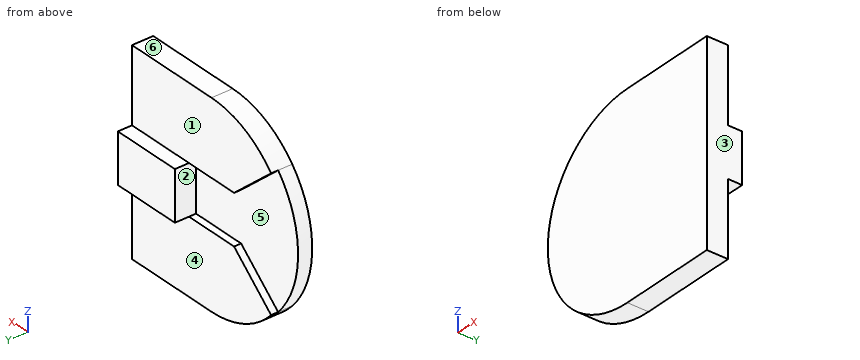
from build123d import *

# Parameters (mm, degrees)
BOSS_EXTRUDE2_DEPTH = 2
BOSS_EXTRUDE3_DEPTH = 3
BOSS_EXTRUDE5_DEPTH = 5


with BuildPart() as part:
    # Sketch1 → Boss-Extrude2 (new body)
    with BuildSketch(Plane(origin=(0, 0, 0), x_dir=(1, 0, 0), z_dir=(0, 1, 0))):
        Polygon((-6.445352893, 3.5), (-10.403887085, 3.5), (-10.403887085, 0), align=None)
        Polygon((-6.445352893, -3.5), (-10.403887085, 0), (-6.445352893, 3.5), (-6.445352893, 0), align=None)
        Polygon((-6.445352893, -3.5), (-10.403887085, 0), (-10.403887085, -3.5), align=None)
        Polygon((-10.403887085, 0), (-10.403887085, 3.5), (-14.362421277, 3.5), align=None)
        with BuildLine():
            Line((-14.362421277, 3.5), (-20.861114748, 9.245921608))
            ThreePointArc((-20.861114748, 9.245921608), (-24.362421277, 0), (-20.861114748, -9.245921608))
            Line((-20.861114748, -9.245921608), (-14.362421277, -3.5))
            Line((-14.362421277, -3.5), (-10.403887085, 0))
            Line((-10.403887085, 0), (-14.362421277, 3.5))
        make_face()
        Polygon((-10.403887085, -3.5), (-10.403887085, 0), (-14.362421277, -3.5), align=None)
    extrude(amount=BOSS_EXTRUDE2_DEPTH)

    # Sketch1_5 → Boss-Extrude3 (add)
    with BuildSketch(Plane(origin=(0, 0, 0), x_dir=(1, 0, 0), z_dir=(0, 1, 0))):
        with BuildLine():
            Line((-10.403887085, 3.5), (-10.403887085, 13.958534192))
            ThreePointArc((-10.403887085, 13.958534192), (-16.138918204, 12.725961451), (-20.861114748, 9.245921608))
            Line((-20.861114748, 9.245921608), (-14.362421277, 3.5))
            Line((-14.362421277, 3.5), (-10.403887085, 3.5))
        make_face()
        with BuildLine():
            ThreePointArc((3.108724683, 3.5), (-1.860298638, 11.038467884), (-10.403887085, 13.958534192))
            Line((-10.403887085, 13.958534192), (-10.403887085, 3.5))
            Line((-10.403887085, 3.5), (-6.445352893, 3.5))
            Line((-6.445352893, 3.5), (3.108724683, 3.5))
        make_face()
        with BuildLine():
            Line((3.554647107, 13.958534192), (-10.403887085, 13.958534192))
            ThreePointArc((-10.403887085, 13.958534192), (-1.860298638, 11.038467884), (3.108724683, 3.5))
            Line((3.108724683, 3.5), (3.554647107, 3.5))
            Line((3.554647107, 3.5), (3.554647107, 13.958534192))
        make_face()
        with BuildLine():
            Line((-14.362421277, -3.5), (-20.861114748, -9.245921608))
            ThreePointArc((-20.861114748, -9.245921608), (-16.138918204, -12.725961451), (-10.403887085, -13.958534192))
            Line((-10.403887085, -13.958534192), (-10.403887085, -3.5))
            Line((-10.403887085, -3.5), (-14.362421277, -3.5))
        make_face()
        with BuildLine():
            Line((-6.445352893, -3.5), (-10.403887085, -3.5))
            Line((-10.403887085, -3.5), (-10.403887085, -13.958534192))
            ThreePointArc((-10.403887085, -13.958534192), (-1.860298638, -11.038467884), (3.108724683, -3.5))
            Line((3.108724683, -3.5), (-6.445352893, -3.5))
        make_face()
        with BuildLine():
            ThreePointArc((3.108724683, -3.5), (-1.860298638, -11.038467884), (-10.403887085, -13.958534192))
            Line((-10.403887085, -13.958534192), (3.554647107, -13.958534192))
            Line((3.554647107, -13.958534192), (3.554647107, -3.5))
            Line((3.554647107, -3.5), (3.108724683, -3.5))
        make_face()
    extrude(amount=BOSS_EXTRUDE3_DEPTH)

    # Sketch1_7 → Boss-Extrude5 (add)
    with BuildSketch(Plane(origin=(0, 0, 0), x_dir=(1, 0, 0), z_dir=(0, 1, 0))):
        with BuildLine():
            ThreePointArc((3.554647107, 0), (3.442717736, 1.764146168), (3.108724683, 3.5))
            Line((3.108724683, 3.5), (-6.445352893, 3.5))
            Line((-6.445352893, 3.5), (-6.445352893, 0))
            Line((-6.445352893, 0), (3.554647107, 0))
        make_face()
        with BuildLine():
            Line((3.554647107, 3.5), (3.108724683, 3.5))
            ThreePointArc((3.108724683, 3.5), (3.442717736, 1.764146168), (3.554647107, 0))
            Line((3.554647107, 0), (3.554647107, 3.5))
        make_face()
        with BuildLine():
            ThreePointArc((3.108724683, -3.5), (3.442717736, -1.764146168), (3.554647107, 0))
            Line((3.554647107, 0), (-6.445352893, 0))
            Line((-6.445352893, 0), (-6.445352893, -3.5))
            Line((-6.445352893, -3.5), (3.108724683, -3.5))
        make_face()
        with BuildLine():
            Line((3.554647107, -3.5), (3.554647107, 0))
            ThreePointArc((3.554647107, 0), (3.442717736, -1.764146168), (3.108724683, -3.5))
            Line((3.108724683, -3.5), (3.554647107, -3.5))
        make_face()
    extrude(amount=BOSS_EXTRUDE5_DEPTH)


solid = part.part
Build history of the part. All positions in model axes, mm. Face numbers are marked on the shaded views. A direction names the side the tool comes from. Round coordinates to 2 decimals unless told otherwise and drop trailing zeros. Write each loop counter-clockwise with the first axis right and the second up, starting at its lowest first coordinate (ties: lowest second). Pieces come first, ordered by that corner, then holes. Notation, with made-up numbers: M 24.5,77.5 L 65.5,77.5 A12 cw 65.5,83.5 Z; hole C 50,31 d7. An arc over 180 degrees is marked long. Answer in a Markdown table with one row per item.
1. Saw through at D-D (x = -1). List the corners of the cut face in (y, z).
Geometry check:
| item | result |
|---|---|
| outline | M 0,-13.96 L 3,-13.96 L 3,-3.5 L 5,-3.5 L 5,3.5 L 3,3.5 L 3,13.96 L 0,13.96 Z |
2. Mould opens along Z. For the marked faces 4, 5 and 6 say: +Z half, -Z half, draft (parallel to the pull), parting line (faces both ways), or undercut.
Geometry check:
| item | result |
|---|---|
| face 4 | draft |
| face 5 | undercut |
| face 6 | +Z half |
3. Probe L1, parallel to Z at x = -1.5, y = 4.45; L2, parallel to Y at x = -14.25, z = -4.5; L3, parallel to Y at x = -19.25, z = 7.75. List the from-to ranges inside material, lowest first. Write a range as [from, to].
Geometry check:
| item | result |
|---|---|
| L1 | [-3.5, 3.5] |
| L2 | [0, 3] |
| L3 | [0, 2] |
4. Saw through at C-C (z = -5.5). List the corners of the cut face in (x, y), and give its area (3 significant figures).
Geometry check:
| item | result |
|---|---|
| outline | M -23.23,0 L 3.55,0 L 3.55,3 L -16.62,3 L -16.62,2 L -23.23,2 Z |
| area | 73.8 mm2 |
5. Which spindle directions (+Z, -Z, +X, -X, +Y, -Y) get a long thin tool onto all of the face, cutting with end or side? Do the marked faces 1, 2 and 3. Say none if no direction does.
Geometry check:
| item | result |
|---|---|
| face 1 | +Z, +X, -X, +Y |
| face 2 | -X, +Y |
| face 3 | +Z, -Z, +X, +Y, -Y |
6. Saw through at B-B (y = 1.1). List the corners of the cut face in (x, z).
Geometry check:
| item | result |
|---|---|
| outline | M -10.4,-13.96 L 3.55,-13.96 L 3.55,13.96 L -10.4,13.96 A13.96 ccw Z |
7. Flat gauge pins, fed straight in: P1, Ø1, axis at x = -14, y = 4.5, coming from the +Z side; P2, Ø9, axis at x = -18, z = 3.5, coming from the +Y side; P3, Ø1, axis at x = -2.5, y = 4, coming from the +Z side; P4, Ø1, axis at x = -3.5, y = 4, coming from the -Z side. Where does each tip first touch, or does it go through?
Geometry check:
| item | result |
|---|---|
| P1 | through |
| P2 | y = 3 |
| P3 | z = 3.5 |
| P4 | z = -3.5 |
8. Saw through at A-A (x = -8). List the corners of the cut face in (y, z).
Geometry check:
| item | result |
|---|---|
| outline | M 0,-13.96 L 3,-13.96 L 3,-3.5 L 2,-3.5 L 2,3.5 L 3,3.5 L 3,13.96 L 0,13.96 Z |
